The model under review builds one solid part; all positions refer to its coordinate system, in mm. A direction names the side the tool comes from. Round coordinates to 2 decimals unless told otherwise and drop trailing zeros. Order: outer loops, then holes, each group sorted by start corner. A loop starts at its lowest first (then second) coordinate and runs counter-clockwise, first axis right, second up.
1) Consider section A-A (x = 25.11). Give the boundary of the cut face in (y, z), then the cut area to 3 significant figures.
2) Consider section D-D (x = -19.5). Give the boundary of the cut face in (y, z).
3) Mouldability with a two-part tool opening along Z and no side actions: class faces 4 (the face through (36, 1, 3)), 5 (the face through (-31.2, 3.4, 1.8)), 6 (the face through (11, 15, 6)) as pulls with the +Z half, pulls with the -Z half, needs draft (parallel to the pull), parting line crosses it, or undercut.
4) Consider section B-B (x = -7). Give the boundary of the cut face in (y, z), then the cut area to 3 significant figures.
5) Machinability: for faces 1 (the face through (-30.012, 16.513, 2.805)), 2 (the face through (34, 2.5, 3)), 3 (the face through (-0.1, -16.3, 10)), which of the approach directions +Z, -Z, +X, -X, +Y, -Y give a long, thin tool a straight path to every point of the face, cutting with its end or side? Answer none if there is none.
6) Clearance check with flat-ended pins moving along their axes: P1, Ø3.5, axis at y = 5, z = 3, coming from the -X side; P2, Ø2.5, axis at x = 25.11, y = 15.29, coming from the -Z side; P3, Ø2, axis at y = -8, z = 3, coming from the -X side; P4, Ø5, axis at x = 38, z = 3.5, coming from the -Y side. State where each tip first meets the part, or that it passes through.
7) Consider section C-C (x = 10). Give the boundary of the cut face in (y, z), then the cut area to 3 significant figures.
8) To check wall thickness, follow L1, parallel to Y at x = 25.11, z = 2.6; L2, parallel to Y at x = 35.3, z = 5.25; L3, parallel to Z at x = -31, y = 5. State the ranges of each line that lie inside material, in increasing order.
from build123d import *

# Parameters (mm, degrees)
SKETCH_1_R                  = 16
EXTRUDE_1_DEPTH             = 12
SKETCH_3_R                  = 18
CUT_EXTRUDE_2_DEPTH         = 6
CUT_EXTRUDE_5_DEPTH         = 2
CUT_EXTRUDE_6_REACH         = 62.994
CUT_EXTRUDE_6_END_RADIUS    = 16
HOLE_WIZARD_M3_AT_2_COUNT   = 2
HOLE_WIZARD_M3_AT_2_PITCH   = 23
HOLE_WIZARD_M3_1_AT_2_COUNT = 2
HOLE_WIZARD_M3_1_AT_2_PITCH = 26
SKETCH_11_R                 = 3.5
CUT_EXTRUDE_8_DEPTH         = 47.717234568
SKETCH_12_W                 = 3
SKETCH_12_H                 = 5
CUT_EXTRUDE_9_DEPTH         = 47.717234568
SKETCH_15_R                 = 1.75
CUT_EXTRUDE_10_DEPTH        = 47.717234568
CHAMFER_1_SIZE              = 0.5


# Read off the part's stored shape, not the designer's step: M4
with BuildPart() as part:
    # Эскиз1 → Бобышка-Вытянуть1 (new body)
    with BuildSketch(Plane.XY):
        Polygon((-34.5, 22.5), (12.5, 22.5), (40.5, 22.5), (40.5, -12.5), (18.5, -12.5), (18.5, -21.5), (-18.5, -21.5), (-18.5, -12.5), (-34.5, -12.5), align=None)
        Circle(SKETCH_1_R, mode=Mode.SUBTRACT)
    extrude(amount=EXTRUDE_1_DEPTH)

    # Эскиз3 → Вырез-Вытянуть2 (cut)
    with BuildSketch(Plane.XY.offset(12)):
        Polygon((18.5, -21.5), (18.5, -12.5), (40.5, -12.5), (40.5, 22.5), (-34.5, 22.5), (-34.5, -12.5), (-18.5, -12.5), (-18.5, -21.5), align=None)
        Circle(SKETCH_3_R, mode=Mode.SUBTRACT)
    extrude(amount=-CUT_EXTRUDE_2_DEPTH, mode=Mode.SUBTRACT)

    # Эскиз4 → Вырез-Вытянуть5 (cut)
    with BuildSketch(Plane.XY.offset(12)):
        with BuildLine():
            ThreePointArc((16, 8.246211251), (0, 18), (-16, 8.246211251))
            Line((-16, 8.246211251), (-16, 8.8e-08))
            ThreePointArc((-16, 8.8e-08), (4.4e-08, 16), (16, 0))
            Line((16, 0), (16, 8.246211251))
        make_face()
        with BuildLine():
            ThreePointArc((16, 0), (-4.4e-08, -16), (-16, 8.8e-08))
            Line((-16, 8.8e-08), (-16, -8.246211251))
            ThreePointArc((-16, -8.246211251), (0, -18), (16, -8.246211251))
            Line((16, -8.246211251), (16, 0))
        make_face()
    extrude(amount=-CUT_EXTRUDE_5_DEPTH, mode=Mode.SUBTRACT)

    # Вырез-Вытянуть6: up to this cylinder (the profile starts outside it)
    cut_extrude_6_end = Plane(origin=(0, 0, 0.402223), z_dir=(0, 0, -1)) * Cylinder(CUT_EXTRUDE_6_END_RADIUS, 158.988, mode=Mode.PRIVATE)
    # Эскиз5 → Вырез-Вытянуть6 (cut, up to the surface)
    with BuildSketch(Plane(origin=(0, 22.5, 0), x_dir=(1, 0, 0), z_dir=(0, 1, 0)), mode=Mode.PRIVATE) as cut_extrude_6_sk1:
        with BuildLine():
            Line((-3.872983346, 0), (3.872983346, 0))
            ThreePointArc((3.872983346, 0), (0, -1), (-3.872983346, 0))
        make_face()
    cut_extrude_6_tool1 = extrude(cut_extrude_6_sk1.sketch, amount=-CUT_EXTRUDE_6_REACH, mode=Mode.PRIVATE) - cut_extrude_6_end
    add(cut_extrude_6_tool1.solids().sort_by_distance((0, 22.5, 0.402223))[0], mode=Mode.SUBTRACT)

    # Эскиз7 → Цековка для  M3 (revolve, cut)
    with BuildSketch(Plane(origin=(35.3, 16.5, 6), x_dir=(0, -1, 0), z_dir=(1, 0, 0))):
        Polygon((0, 0), (0, 6), (1.625, 6), (1.6, 5.975), (1.6, 2.525), (1.625, 2.5), (3.25, 2.5), (3.25, 0.025), (3.275, 0), align=None)
    hole_wizard_m3 = revolve(axis=Axis((35.3, 16.5, 12.35), (0, 0, -1)), mode=Mode.SUBTRACT)

    # Цековка для  M3 at 2: Цековка для  M3 ×2
    with Locations(*[(0, -i * HOLE_WIZARD_M3_AT_2_PITCH, 0) for i in range(1, HOLE_WIZARD_M3_AT_2_COUNT)]):
        add(hole_wizard_m3, mode=Mode.SUBTRACT)

    # Эскиз9 → M3_1 (revolve, cut)
    with BuildSketch(Plane(origin=(-34.5, -8, 3), x_dir=(0, 0, 1), z_dir=(0, 1, 0))):
        Polygon((0, 0), (0, 12.251075774), (1.25, 11.5), (1.25, 9), (1.5, 9), (1.5, 0.1), (1.6, 0), align=None)
    hole_wizard_m3_1 = revolve(axis=Axis((-40.85, -8, 3), (1, 0, 0)), mode=Mode.SUBTRACT)

    # M3_1 at 2: M3_1 ×2
    with Locations(*[(0, i * HOLE_WIZARD_M3_1_AT_2_PITCH, 0) for i in range(1, HOLE_WIZARD_M3_1_AT_2_COUNT)]):
        add(hole_wizard_m3_1, mode=Mode.SUBTRACT)

    # Эскиз11 → Вырез-Вытянуть8 (cut, through all)
    with BuildSketch(Plane.XY.offset(6)):
        with Locations((-24.5, 5)):
            Circle(SKETCH_11_R)
    extrude(amount=-CUT_EXTRUDE_8_DEPTH, mode=Mode.SUBTRACT)

    # Эскиз12 → Вырез-Вытянуть9 (cut, through all)
    with BuildSketch(Plane.XY.offset(6)):
        Polygon((40.5, 0), (40.5, 10), (36, 10), (36, 7.5), (36, 2.5), (36, 0), align=None)
        with Locations((34.5, 5)):
            Rectangle(SKETCH_12_W, SKETCH_12_H)
    extrude(amount=-CUT_EXTRUDE_9_DEPTH, mode=Mode.SUBTRACT)

    # M4 outline → M4 (revolve, cut)
    with BuildSketch(Plane(origin=(0, 5, 3), x_dir=(0, 1, 0), z_dir=(0, 0, -1))):
        Polygon((2.275, -28), (2.275, -27.159503456), (0, -27.159503456), (0, -34.5), (2.275, -34.5), (2, -34.225), (2, -28.275), align=None)
    revolve(axis=Axis((0, 5, 3), (1, 0, 0)), mode=Mode.SUBTRACT)

    # Эскиз15 → Вырез-Вытянуть10 (cut, through all)
    with BuildSketch(Plane.XY.offset(6)):
        with Locations((25.11, 10.285533906)):
            Circle(SKETCH_15_R)
    extrude(amount=-CUT_EXTRUDE_10_DEPTH, mode=Mode.SUBTRACT)

    # Эскиз16 → M3_2 (revolve, cut)
    with BuildSketch(Plane(origin=(25.11, 15.285533906, 6), x_dir=(0, -1, 0), z_dir=(1, 0, 0))):
        Polygon((0, 0), (0, 6), (1.7, 6), (1.5, 5.8), (1.5, 0.2), (1.7, 0), align=None)
    revolve(axis=Axis((25.11, 15.285533906, 12.35), (0, 0, -1)), mode=Mode.SUBTRACT)

    # Фаска1
    chamfer_1_edges = [part.edges().sort_by_distance(p)[0] for p in [
        (-18, 0, 12),
        (17.492855685, -4.242640687, 12),
    ]]
    chamfer(chamfer_1_edges, length=CHAMFER_1_SIZE)


solid = part.part
Answer below:
1. outline: (-12.5, 0) - (8.54, 0) - (8.54, 6) - (-12.5, 6) - close; (12.04, 0) - (13.59, 0) - (13.79, 0.2) - (13.79, 5.8) - (13.59, 6) - (12.04, 6) - close; (16.79, 0.2) - (16.99, 0) - (22.5, 0) - (22.5, 6) - (16.99, 6) - (16.79, 5.8) - close
1. area: 171 mm2
2. outline: (-12.5, 0) - (22.5, 0) - (22.5, 6) - (-12.5, 6) - close
3. face 4: needs draft
3. face 5: undercut
3. face 6: pulls with the +Z half
4. outline: (-21.5, 0) - (-14.39, 0) - (-14.39, 10) - (-16.58, 10) - (-16.58, 6) - (-21.5, 6) - close; (14.39, 0) - (22.5, 0) - (22.5, 6) - (16.58, 6) - (16.58, 10) - (14.39, 10) - close
4. area: 109 mm2
5. face 1: -X
5. face 2: +Z, -Z, +X
5. face 3: +Z, +Y, -Y
6. P1: stops at x = -21.47
6. P2: passes through
6. P3: stops at x = -22.85
6. P4: stops at y = -12.5
7. outline: (-21.5, 0) - (-12.49, 0) - (-12.49, 10) - (-14.97, 10) - (-14.97, 6) - (-21.5, 6) - close; (12.49, 0) - (22.5, 0) - (22.5, 6) - (14.97, 6) - (14.97, 10) - (12.49, 10) - close
7. area: 134 mm2
8. L1: y = -12.5 to 8.54, 12.04 to 13.79, 16.79 to 22.5
8. L2: y = -12.5 to -9.75, -3.25 to 2.5, 7.5 to 13.25, 19.75 to 22.5
8. L3: z = 0 to 1, 5 to 6
